Model file for the job. Use its own axes, mm. A direction names the side the tool comes from. Give positions to 0.01 mm unless a question says otherwise; leave off trailing zeros. Loops run counter-clockwise (first coordinate to the right, second up) from the corner with the lowest first, then second, coordinate; pieces in that order, holes last. Notation, with made-up numbers: M 34,3.5 L 45,3.5 A7 ccw 45,11.5 Z; hole C 49,-2 d6. An arc over 180 degrees is marked long. Answer in a Markdown table with one row per item.
```python
from build123d import *

# Parameters (mm, degrees)
SKIZZE1_W                       = 48.5
SKIZZE1_H                       = 38
AUFSATZ_LINEAR_AUSTRAGEN1_DEPTH = 2
SKIZZE2_R                       = 1.5
SKIZZE2_R_2                     = 2.5
AUFSATZ_LINEAR_AUSTRAGEN2_DEPTH = 3
SKIZZE3_R                       = 1.4
SKIZZE3_R_2                     = 0.9
AUFSATZ_LINEAR_AUSTRAGEN3_DEPTH = 3


with BuildPart() as part:
    # Skizze1 → Aufsatz-Linear austragen1 (new body)
    with BuildSketch(Plane(origin=(0, 0, 0), x_dir=(0, 1, 0), z_dir=(0, 0, 1))):
        Rectangle(SKIZZE1_W, SKIZZE1_H)
    extrude(amount=AUFSATZ_LINEAR_AUSTRAGEN1_DEPTH)

    # Skizze2 → Aufsatz-Linear austragen2 (add)
    with BuildSketch(Plane.XY.offset(2)):
        with Locations((-16, -22.25)):
            Circle(SKIZZE2_R)
        with Locations((16, -22.25)):
            Circle(SKIZZE2_R)
        with Locations(Location((16, 22.75, 0), (0, 0, 90))):
            Circle(SKIZZE2_R)
        with Locations(Location((-16, 22.75, 0), (0, 0, 90))):
            Circle(SKIZZE2_R)
        with Locations((0, 20.75)):
            Circle(SKIZZE2_R_2)
        with Locations((0, -20.75)):
            Circle(SKIZZE2_R_2)
    extrude(amount=AUFSATZ_LINEAR_AUSTRAGEN2_DEPTH)

    # Skizze3 → Aufsatz-Linear austragen3 (add)
    with BuildSketch(Plane.XY.offset(5)):
        with Locations((0, 20.75)):
            Circle(SKIZZE3_R)
        with Locations((16, 22.75)):
            Circle(SKIZZE3_R_2)
        with Locations((-16, 22.75)):
            Circle(SKIZZE3_R_2)
        with Locations((0, -20.75)):
            Circle(SKIZZE3_R)
        with Locations((-16, -22.25)):
            Circle(SKIZZE3_R_2)
        with Locations((16, -22.25)):
            Circle(SKIZZE3_R_2)
    extrude(amount=AUFSATZ_LINEAR_AUSTRAGEN3_DEPTH)


solid = part.part
```
(1) Flat gauge pins, fed straight in: P1, Ø6, axis at x = -4, y = -2, coming from the +Z side; P2, Ø1, axis at y = -10.5, z = 3, coming from the +X side. Where does each tip first touch, or does it go through?
Established:
| item | result |
|---|---|
| P1 | stops at z = 2 |
| P2 | passes through |
(2) Saw through at B-B, the plane y = -5. Give the cut face in (x, z).
Established:
| item | result |
|---|---|
| outline | M -19,0 L 19,0 L 19,2 L -19,2 Z |
(3) Saw through at C-C, the plane x = -10.5. Give the cut face in (y, z), and give its area (3 significant figures).
Established:
| item | result |
|---|---|
| outline | M -24.25,0 L 24.25,0 L 24.25,2 L -24.25,2 Z |
| area | 97.0 mm2 |
(4) Saw through at A-A, the plane x = 0. Give the cut face in (y, z), and give its area (3 significant figures).
Established:
| item | result |
|---|---|
| outline | M -24.25,0 L 24.25,0 L 24.25,2 L 23.25,2 L 23.25,5 L 22.15,5 L 22.15,8 L 19.35,8 L 19.35,5 L 18.25,5 L 18.25,2 L -18.25,2 L -18.25,5 L -19.35,5 L -19.35,8 L -22.15,8 L -22.15,5 L -23.25,5 L -23.25,2 L -24.25,2 Z |
| area | 144 mm2 |
(5) Which spindle directions (+Z, -Z, +X, -X, +Y, -Y) get a long thin tool onto all of the face, cutting with end or side? Do faces 1 (the flat face through (-19, 0, 1)), 2 (the cylindrical face through (1.34, -18.64, 3.48)). Say none if no direction does.
Established:
| item | result |
|---|---|
| face 1 | +Z, -Z, -X, +Y, -Y |
| face 2 | +Z |
(6) Wall check: L1, parallel to Z at x = -5.5, y = 3.5; L2, parallel to Y at x = 16.5, z = 4; L3, parallel to X at y = 21, z = 3. Give the ranges that are in metal, low to high.
Established:
| item | result |
|---|---|
| L1 | z = 0 to 2 |
| L2 | y = -23.66 to -20.84, 21.34 to 24.16 |
| L3 | x = -2.49 to 2.49 |
(7) Mould opens along Y. For faces 3 (the flat face through (0, -21, 8)), 4 (the cylindrical face through (-17.11, -21.24, 3.48)), 5 (the flat face through (0, -24.25, 1)) say: pulls with the +Y half, pulls with the -Y half, needs draft (parallel to the pull), parting line crosses it, or undercut.
Established:
| item | result |
|---|---|
| face 3 | needs draft |
| face 4 | undercut |
| face 5 | pulls with the -Y half |
